```python
from build123d import *

# Parameters (mm, degrees)
BOSS_EXTRUDE1_DEPTH   = 3
BOSS_EXTRUDE1_2_DEPTH = 3
BOSS_EXTRUDE1_3_DEPTH = 3
BOSS_EXTRUDE1_4_DEPTH = 3
BOSS_EXTRUDE2_DEPTH   = 20
SKETCH3_W             = 24
SKETCH3_H             = 13
SKETCH3_R             = 6
SKETCH3_R_2           = 0.75
SKETCH3_R_3           = 0.8
CUT_EXTRUDE1_DEPTH    = 207
SKETCH4_W             = 24
SKETCH4_H             = 13
SKETCH4_R             = 6
SKETCH4_R_2           = 0.75
CUT_EXTRUDE3_DEPTH    = 157


with BuildPart() as part:
    # Sketch1 → Boss-Extrude1 (new body)
    with BuildSketch(Plane(origin=(0, 0, 0), x_dir=(1, 0, 0), z_dir=(0, 1, 0))):
        with BuildLine():
            ThreePointArc((-64, 84), (-95.819805153, 70.819805153), (-109, 39))
            Line((-109, 39), (-94, 39))
            ThreePointArc((-94, 39), (-85.213203436, 60.213203436), (-64, 69))
            Line((-64, 69), (-64, 84))
        make_face()
    extrude(amount=-BOSS_EXTRUDE1_DEPTH)



with BuildPart() as body_2:
    # Sketch1 → Boss-Extrude1 2 (new body)
    with BuildSketch(Plane(origin=(0, 0, 0), x_dir=(1, 0, 0), z_dir=(0, 1, 0))):
        with BuildLine():
            ThreePointArc((109, 39), (95.819805153, 70.819805153), (64, 84))
            Line((64, 84), (64, 69))
            ThreePointArc((64, 69), (85.213203436, 60.213203436), (94, 39))
            Line((94, 39), (109, 39))
        make_face()
    extrude(amount=-BOSS_EXTRUDE1_2_DEPTH)


with BuildPart() as body_3:
    # Sketch1 → Boss-Extrude1 3 (new body)
    with BuildSketch(Plane(origin=(0, 0, 0), x_dir=(1, 0, 0), z_dir=(0, 1, 0))):
        with BuildLine():
            ThreePointArc((-109, -39), (-95.819805153, -70.819805153), (-64, -84))
            Line((-64, -84), (-64, -69))
            ThreePointArc((-64, -69), (-85.213203436, -60.213203436), (-94, -39))
            Line((-94, -39), (-109, -39))
        make_face()
    extrude(amount=-BOSS_EXTRUDE1_3_DEPTH)


with BuildPart() as body_4:
    # Sketch1 → Boss-Extrude1 4 (new body)
    with BuildSketch(Plane(origin=(0, 0, 0), x_dir=(1, 0, 0), z_dir=(0, 1, 0))):
        with BuildLine():
            ThreePointArc((64, -84), (95.819805153, -70.819805153), (109, -39))
            Line((109, -39), (94, -39))
            ThreePointArc((94, -39), (85.213203436, -60.213203436), (64, -69))
            Line((64, -69), (64, -84))
        make_face()
    extrude(amount=-BOSS_EXTRUDE1_4_DEPTH)


with BuildPart() as part_1:
    add(part.part)

    add(body_2.part)  # Boss-Extrude2 merges body 2

    add(body_3.part)  # Boss-Extrude2 merges body 3

    add(body_4.part)  # Boss-Extrude2 merges body 4
    # Sketch1<6> → Boss-Extrude2 (add)
    with BuildSketch(Plane(origin=(0, 0, 0), x_dir=(1, 0, 0), z_dir=(0, 1, 0))):
        with BuildLine():
            Line((-64, 78.5), (64, 78.5))
            ThreePointArc((64, 78.5), (91.930717857, 66.930717857), (103.5, 39))
            Line((103.5, 39), (103.5, -39))
            ThreePointArc((103.5, -39), (91.930717857, -66.930717857), (64, -78.5))
            Line((64, -78.5), (-64, -78.5))
            ThreePointArc((-64, -78.5), (-91.930717857, -66.930717857), (-103.5, -39))
            Line((-103.5, -39), (-103.5, 39))
            ThreePointArc((-103.5, 39), (-91.930717857, 66.930717857), (-64, 78.5))
        make_face()
        with BuildLine():
            Line((-64, 74.5), (64, 74.5))
            ThreePointArc((64, 74.5), (89.102290732, 64.102290732), (99.5, 39))
            Line((99.5, 39), (99.5, -39))
            ThreePointArc((99.5, -39), (89.102290732, -64.102290732), (64, -74.5))
            Line((64, -74.5), (-64, -74.5))
            ThreePointArc((-64, -74.5), (-89.102290732, -64.102290732), (-99.5, -39))
            Line((-99.5, -39), (-99.5, 39))
            ThreePointArc((-99.5, 39), (-89.102290732, 64.102290732), (-64, 74.5))
        make_face(mode=Mode.SUBTRACT)
    extrude(amount=BOSS_EXTRUDE2_DEPTH)

    # Sketch3 → Cut-Extrude1 (cut)
    with BuildSketch(Plane.ZY.offset(103.5)):
        with Locations((-5.5, 10)):
            Rectangle(SKETCH3_W, SKETCH3_H)
        with Locations((0, 10)):
            Circle(SKETCH3_R, mode=Mode.SUBTRACT)
        with Locations((-19.5, 10)):
            Circle(SKETCH3_R_2)
        with Locations((0, 10)):
            Circle(SKETCH3_R)
        with Locations((8.5, 10)):
            Circle(SKETCH3_R_3)
    extrude(amount=-CUT_EXTRUDE1_DEPTH, mode=Mode.SUBTRACT)

    # Sketch4 → Cut-Extrude3 (cut)
    with BuildSketch(Plane.XY.offset(78.5)):
        with Locations((-5.5, 10)):
            Rectangle(SKETCH4_W, SKETCH4_H)
        with Locations((0, 10)):
            Circle(SKETCH4_R, mode=Mode.SUBTRACT)
        with Locations((-19.15, 10.35)):
            Circle(SKETCH4_R_2)
        with Locations((8.15, 10.35)):
            Circle(SKETCH4_R_2)
        with Locations((0, 10)):
            Circle(SKETCH4_R)
    extrude(amount=-CUT_EXTRUDE3_DEPTH, mode=Mode.SUBTRACT)


solid = part_1.part
```
The listing builds one solid part. Answer for the finished solid, in the listing's coordinates (mm). A direction names the side the tool comes from. Round coordinates to 2 decimals unless told otherwise and drop trailing zeros. Loops run counter-clockwise (first coordinate to the right, second up) from the corner with the lowest first, then second, coordinate; pieces in that order, holes last. Notation, with made-up numbers: (19.25, 24.5) -> (77.25, 24.5) arc R14 cw to (77.25, 32.5) -> close; hole circle Ø4 at (15.5, 54). An arc over 180 degrees is marked (long way). Use one line per item in the form item = value.
1. The part is cut by section C-C on x = 2. Determine the outline of the cut face in (y, z).
Answer key:
outline = (0, -78.5) -> (3.5, -78.5) -> (3.5, -74.5) -> (0, -74.5) -> close; (0, 74.5) -> (3.5, 74.5) -> (3.5, 78.5) -> (0, 78.5) -> close; (16.5, -78.5) -> (20, -78.5) -> (20, -74.5) -> (16.5, -74.5) -> close; (16.5, 74.5) -> (20, 74.5) -> (20, 78.5) -> (16.5, 78.5) -> close
2. A tool of negligible diameter and unlimited length cuts with its end or side. For faces 4 (the flat face through (86, -3, 61)), 5 (the cylindrical face through (-92.24, 9.86, -66.62)), 6 (the flat face through (-1, 3, -74.5)), 7 (the flat face through (-86, 0, -61)), 8 (the cylindrical face through (91.62, 9.86, -67.24)), from which of +Z, -Z, +X, -X, +Y, -Y can it reach the whole face along a straight path? Write none if from no direction.
Answer key:
face_4 = +Z, -Z, +X, -X, -Y
face_5 = -Z, -X, +Y
face_6 = +Y, -Y
face_7 = +Y
face_8 = -Z, +X, +Y
3. Find the intervals of material crossed by probe 1 along Z at (x, y) = (28, 12); probe 2 along X at (y, z) = (14.5, -32); probe 3 along Y at (x, z) = (100.45, -19.5), in increasing order. Write a range as [from, to].
Answer key:
probe_1 = [-78.5, -74.5], [74.5, 78.5]
probe_2 = [-103.5, -99.5], [99.5, 103.5]
probe_3 = [0, 9.25], [10.75, 20]
4. For a pull along X with two mould halves and no side action, classify faces 1 (the cylindrical face through (-89.4, 9.9, -63.8)), 2 (the flat face through (103.5, 3, -1)), 3 (the flat face through (-103.5, 3, 1)) as released by +X, released by -X, zero draft, split by the parting line, or undercut.
Answer key:
face_1 = undercut
face_2 = released by +X
face_3 = released by -X
5. The part is cut by section A-A on z = 32. Determine the outline of the cut face in (x, y).
Answer key:
outline = (-103.5, 0) -> (-99.5, 0) -> (-99.5, 20) -> (-103.5, 20) -> close; (99.5, 0) -> (103.5, 0) -> (103.5, 20) -> (99.5, 20) -> close
6. The part is cut by section D-D on z = -11.5. Determine the outline of the cut face in (x, y).
Answer key:
outline = (-103.5, 0) -> (-99.5, 0) -> (-99.5, 3.5) -> (-103.5, 3.5) -> close; (-103.5, 16.5) -> (-99.5, 16.5) -> (-99.5, 20) -> (-103.5, 20) -> close; (99.5, 0) -> (103.5, 0) -> (103.5, 3.5) -> (99.5, 3.5) -> close; (99.5, 16.5) -> (103.5, 16.5) -> (103.5, 20) -> (99.5, 20) -> close
7. Flat-ended cylindrical pins translate along their axes: pin 1 Ø3 at (x, z) = (-101.5, -9) entering from -Y; pin 2 Ø13.5 at (x, z) = (-92.5, -55.5) entering from +Y; pin 3 Ø2.5 at (y, z) = (-2, -79.5) entering from +X; pin 4 Ø2 at (x, y) = (-25.5, 15.5) entering from -Z. Find the tip coordinate at first contact, or state that the pin passes through.
Answer key:
pin_1 = 0
pin_2 = 20
pin_3 = 86.01
pin_4 = -78.5
8. The part is cut by section B-B on x = 45.5. Determine the outline of the cut face in (y, z).
Answer key:
outline = (0, -78.5) -> (20, -78.5) -> (20, -74.5) -> (0, -74.5) -> close; (0, 74.5) -> (20, 74.5) -> (20, 78.5) -> (0, 78.5) -> close
